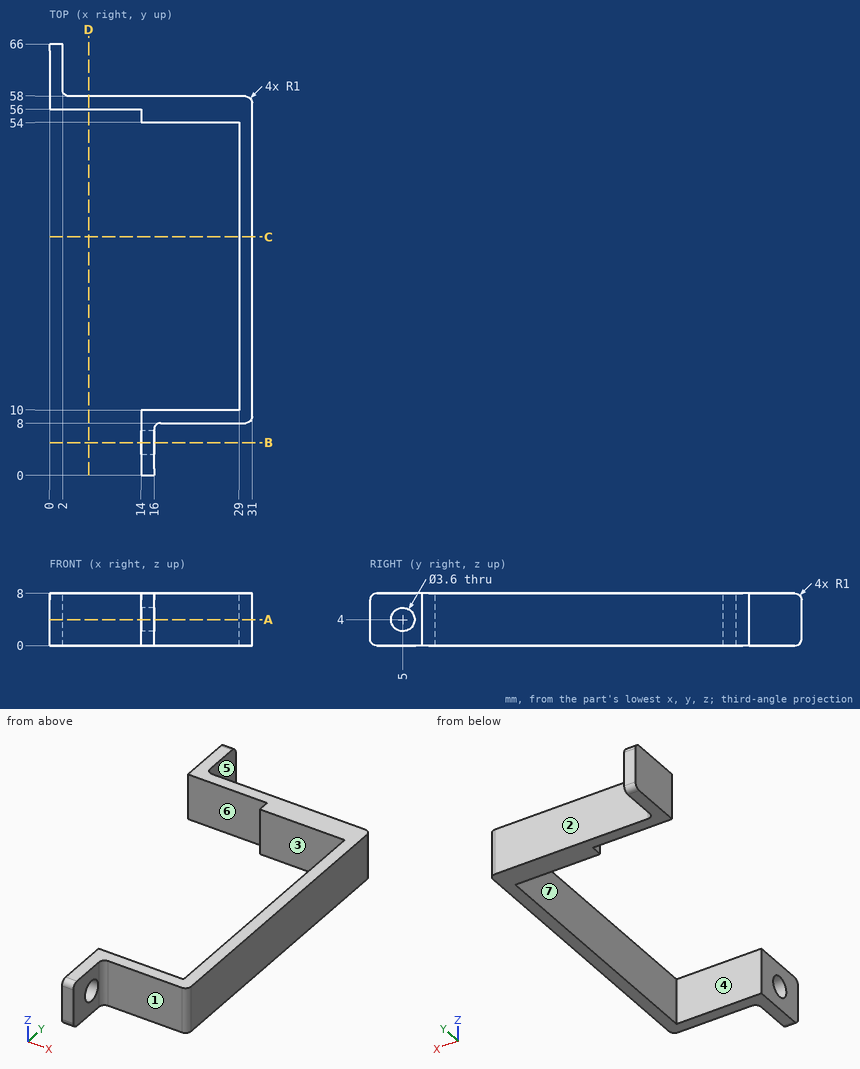
Geometry: see drawing. Coordinates: mm, zero at the bounding-box minimum. A direction names the side the tool comes from. Coordinates: 2 decimals unless noted, no trailing zeros. Order: outer loops, then holes, each group sorted by start corner. A loop starts at its lowest first (then second) coordinate and runs counter-clockwise, first axis right, second up. Notation, with made-up numbers: M 81.25,52 L 99.25,52 A8 ccw 99.25,56 Z; hole C 28,-28.75 d8. An arc over 180 degrees is marked long. Answer in a Markdown table with one row per item. Add a question column.
Q1. Line query: L1, parallel to Y at x = 28.5, z = 6; L2, parallel to Y at x = 10.5, z = 7.25; L3, parallel to Z at x = 15.1, y = 5. Output: solid intervals per line, ascending.
Q2. Section query C-C on y = 36.5. Return the cut outline in (x, z).
Q3. Section query D-D on x = 6. Return the cut outline in (y, z), and give its area (3 significant figures).
Q4. Section query A-A on z = 4. Return the cut outline in (x, y).
Q5. Contact query for flat-ended pins moving along their axis: P1, Ø1, axis at y = 55, z = 2.5, coming from the -X side; P2, Ø4, axis at x = 22.5, z = 1.5, coming from the -Y side; P3, Ø1.5, axis at x = 26, z = 7, coming from the +Y side; P4, Ø3, axis at y = 5, z = 4, coming from the +X side. Output: stop coordinate, or through.
Q6. Section query B-B on y = 5. Return the cut outline in (x, z).
Q7. Mould query, pull axis Y, two halves, no side actions, for the marked faces 1, 2, 3 and 4. Classes: released by +Y, released by -Y, zero draft, split by the parting line, or undercut.
Q8. Reachability of the marked faces 5, 6 and 7 from +Z, -Z, +X, -X, +Y, -Y: full face, straight path, thin tool, end or side. Return the list, or none.
Completed:
| question | item | result |
|---|---|---|
| 1 | L1 | y = 8 to 10, 54 to 58 |
| 1 | L2 | y = 56 to 58 |
| 1 | L3 | z = 0 to 2.2, 5.8 to 8 |
| 2 | outline | M 29,0 L 31,0 L 31,8 L 29,8 Z |
| 3 | outline | M 56,0 L 58,0 L 58,8 L 56,8 Z |
| 3 | area | 16.0 mm2 |
| 4 | outline | M 0,56 L 14,56 L 14,54 L 29,54 L 29,10 L 14,10 L 14,6.8 L 16,6.8 L 16,7 A1 cw 17,8 L 30,8 A1 ccw 31,9 L 31,57 A1 ccw 30,58 L 3,58 A1 cw 2,59 L 2,66 L 0,66 Z; M 14,0 L 16,0 L 16,3.2 L 14,3.2 Z |
| 5 | P1 | stops at x = 14 |
| 5 | P2 | stops at y = 8 |
| 5 | P3 | stops at y = 58 |
| 5 | P4 | passes through |
| 6 | outline | M 14,0 L 16,0 L 16,2.2 L 14,2.2 Z; M 14,5.8 L 16,5.8 L 16,8 L 14,8 Z |
| 7 | face 1 | released by -Y |
| 7 | face 2 | released by +Y |
| 7 | face 3 | undercut |
| 7 | face 4 | undercut |
| 8 | face 5 | +Z, -Z, +X, +Y |
| 8 | face 6 | +Z, -Z, -X, -Y |
| 8 | face 7 | +Z, -Z, -X |
